from build123d import *

# Parameters (mm, degrees)
SKETCH1_W           = 165
SKETCH1_H           = 30
BOSS_EXTRUDE1_DEPTH = 2
FILLET1_R           = 5
SKETCH3_R           = 4
SKETCH3_R_2         = 1.5
CUT_EXTRUDE1_DEPTH  = 2
SKETCH4_R           = 7.5
CUT_EXTRUDE2_DEPTH  = 10
SKETCH5_R           = 1.5
CUT_EXTRUDE3_DEPTH  = 10
SKETCH6_R           = 1.5
CUT_EXTRUDE4_DEPTH  = 84.876397157


with BuildPart() as part:
    # Sketch1 → Boss-Extrude1 (new body)
    with BuildSketch(Plane(origin=(0, 0, 0), x_dir=(1, 0, 0), z_dir=(0, 1, 0))):
        Rectangle(SKETCH1_W, SKETCH1_H)
    extrude(amount=BOSS_EXTRUDE1_DEPTH)

    # Fillet1
    fillet1_edges = [part.edges().sort_by_distance(p)[0] for p in [
        (82.5, 1, 15),
        (-82.5, 1, 15),
        (-82.5, 1, -15),
        (82.5, 1, -15),
    ]]
    fillet(fillet1_edges, radius=FILLET1_R)

    # Sketch3 → Cut-Extrude1 (cut)
    with BuildSketch(Plane(origin=(0, 2, 0), x_dir=(1, 0, 0), z_dir=(0, 1, 0))):
        with Locations(Location((-67.5, 0, 0), (0, 0, 270))):
            Circle(SKETCH3_R)
        with Locations(Location((-67.5, 7.5, 0), (0, 0, 270))):
            Circle(SKETCH3_R_2)
        with Locations(Location((-61.555061089, -4.572493996, 0), (0, 0, 270))):
            Circle(SKETCH3_R_2)
        with Locations(Location((-73.130988244, -4.953985406, 0), (0, 0, 270))):
            Circle(SKETCH3_R_2)
    extrude(amount=-CUT_EXTRUDE1_DEPTH, mode=Mode.SUBTRACT)

    # Sketch4 → Cut-Extrude2 (cut)
    with BuildSketch(Plane(origin=(0, 2, 0), x_dir=(1, 0, 0), z_dir=(0, 1, 0))):
        with Locations((82.5, 0)):
            Circle(SKETCH4_R)
    extrude(amount=-CUT_EXTRUDE2_DEPTH, mode=Mode.SUBTRACT)

    # Sketch5 → Cut-Extrude3 (cut)
    with BuildSketch(Plane(origin=(0, 2, 0), x_dir=(1, 0, 0), z_dir=(0, 1, 0))):
        with Locations(Location((-32.5, 10, 0), (0, 0, 270))):
            Circle(SKETCH5_R)
        with Locations(Location((37.5, 10, 0), (0, 0, 270))):
            Circle(SKETCH5_R)
        with Locations(Location((-32.5, -10, 0), (0, 0, 270))):
            Circle(SKETCH5_R)
        with Locations(Location((37.5, -10, 0), (0, 0, 270))):
            Circle(SKETCH5_R)
    extrude(amount=-CUT_EXTRUDE3_DEPTH, mode=Mode.SUBTRACT)

    # Sketch6 → Cut-Extrude4 (cut, through all)
    with BuildSketch(Plane(origin=(0, 2, 0), x_dir=(1, 0, 0), z_dir=(0, 1, 0))):
        with Locations(Location((72.5, 10, 0), (0, 0, 270))):
            Circle(SKETCH6_R)
        with Locations(Location((72.5, -10, 0), (0, 0, 270))):
            Circle(SKETCH6_R)
    extrude(amount=-CUT_EXTRUDE4_DEPTH, mode=Mode.SUBTRACT)


solid = part.part
The model under review builds one solid part; all positions refer to its coordinate system, in mm. Round coordinates to 2 decimals unless told otherwise and drop trailing zeros. Write each loop counter-clockwise with the first axis right and the second up, starting at its lowest first coordinate (ties: lowest second). Pieces come first, ordered by that corner, then holes. Notation, with made-up numbers: M 27,34 L 41,34 A27 ccw 41,62 Z; hole C -29.5,3.5 d4. An arc over 180 degrees is marked long. Use a Markdown table: item, result. Add a question column.
Q1. To check wall thickness, follow line 1 (X direction, y = 0.2, z = 10.25); line 2 (Z direction, x = 72.5, y = 0.85); line 3 (X direction, y = 1.15, z = -11.25). State the ranges of each line that lie inside material, in increasing order.
Q2. We need section C-C, the plane y = 0.6. Count the separate pieces of the cut face and the enclosed holes in it, plus the area to 3 significant figures.
Q3. We need section A-A, the plane x = -67.5. State the section outline as (y, z) points, plus the area to 3 significant figures.
Q4. We need section B-B, the plane z = 0. State the section outline as (x, y) points.
Q5. The part is to be moulded in two halves that separate along Z. For faces 1 (the face through (81.07, 1.01, -13.5)), 2 (the face through (-66.013, 1.014, -7.695)), 3 (the face through (75, 1, 0)), 4 (the face through (-1, 0, 0)), say which applies: pulls with the +Z half, pulls with the -Z half, needs draft (parallel to the pull), parting line crosses it, or undercut.
Q6. We need section D-D, the plane x = 72.5. State the section outline as (y, z) points.
Findings below:
| question | item | result |
|---|---|---|
| 1 | line 1 | x = -82.49 to -33.98, -31.02 to 36.02, 38.98 to 71.02, 73.98 to 82.49 |
| 1 | line 2 | z = -15 to -11.5, -8.5 to 8.5, 11.5 to 15 |
| 1 | line 3 | x = -82.34 to -33.33, -31.67 to 36.67, 38.33 to 71.67, 73.33 to 82.34 |
| 2 | separate pieces | 1 |
| 2 | enclosed holes | 10 |
| 2 | area | 4,730 mm² |
| 3 | outline | M 0,-15 L 2,-15 L 2,-9 L 0,-9 Z; M 0,-6 L 2,-6 L 2,-4 L 0,-4 Z; M 0,4 L 2,4 L 2,15 L 0,15 Z |
| 3 | area | 38.0 mm² |
| 4 | outline | M -82.5,0 L -71.5,0 L -71.5,2 L -82.5,2 Z; M -63.5,0 L 75,0 L 75,2 L -63.5,2 Z |
| 5 | face 1 | pulls with the -Z half |
| 5 | face 2 | undercut |
| 5 | face 3 | undercut |
| 5 | face 4 | needs draft |
| 6 | outline | M 0,-15 L 2,-15 L 2,-11.5 L 0,-11.5 Z; M 0,-8.5 L 2,-8.5 L 2,8.5 L 0,8.5 Z; M 0,11.5 L 2,11.5 L 2,15 L 0,15 Z |
